Autodesk Inventor part; units mm, degrees
ref_plane "YZ Plane" through (0, 0, 0) normal (1, 0, 0) x (0, 1, 0)
ref_plane "XZ Plane" through (0, 0, 0) normal (0, 1, 0) x (-1, 0, 0)
ref_plane "XY Plane" through (0, 0, 0) normal (0, 0, 1) x (1, 0, 0)
sketch "Skizze1" plane through (0, 0, 0) normal (0, 1, 0) x (-1, 0, 0)
  line L0 (-60, -60) -> (60, -60)
  line L1 (60, -60) -> (60, 60)
  line L2 (60, 60) -> (-60, 60)
  line L3 (-60, 60) -> (-60, -60)
  line L4 (-60, -60) -> (60, 60) construction
  line L5 (60, -60) -> (-60, 60) construction
  point P0 (0, 0)
  dimension "d0" = 120
  dimension "d1" = 120
extrude "Extrusion1" add sketch "Skizze1" along normal blind 25
sketch "Skizze2" plane through (0, 25, 0) normal (0, 1, 0) x (1, 0, 0)
  line L0 (52.5, 52.5) -> (-52.5, 52.5)
  line L1 (-52.5, 52.5) -> (-52.5, -52.5)
  line L2 (-52.5, -52.5) -> (52.5, -52.5)
  line L3 (52.5, -52.5) -> (52.5, 52.5)
  line L4 (52.5, 52.5) -> (-52.5, -52.5) construction
  line L5 (-52.5, 52.5) -> (52.5, -52.5) construction
  point P0 (0, 0)
  dimension "d4" = 105
  dimension "d5" = 105
hole "Bohrung1" at (52.5, 25, 52.5) at (52.5, 25, -52.5) at (-52.5, 25, 52.5) at (-52.5, 25, -52.5) direction (0, -1, 0) diameter 4.3 end through all
sketch "Skizze3" plane through (0, 25, 0) normal (0, 1, 0) x (1, 0, 0)
  circle A0 centre (0, 0) radius 56.5
  dimension "d13" = 113
extrude "Extrusion2" cut sketch "Skizze3" against normal through all
fillet "Rundung1" radius 2 4 edges at (-60, 12.5, 60) (60, 12.5, 60) (-60, 12.5, -60) (60, 12.5, -60)
properties part number "Lüfter80x80"
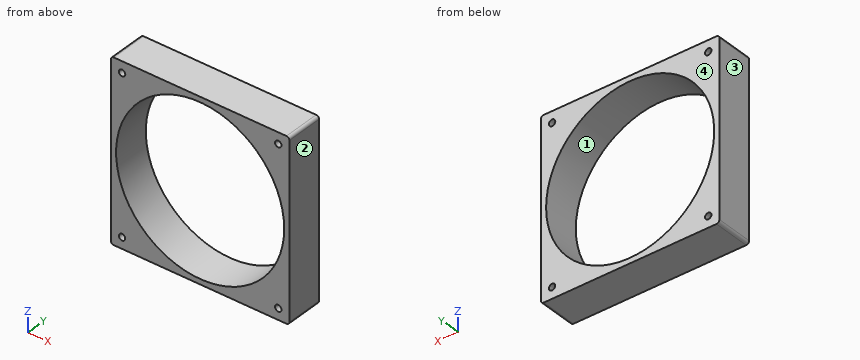
CAD build for the part. Positions are in the model's coordinates, mm. Face numbers are marked on the shaded views. Round coordinates to 2 decimals unless told otherwise and drop trailing zeros. Order: outer loops, then holes, each group sorted by start corner. A loop starts at its lowest first (then second) coordinate and runs counter-clockwise, first axis right, second up. Notation, with made-up numbers: (24, 42.5) - (43, 42.5) arc R13 cw to (43, 49.5) - close; hole circle Ø11 at (74, 72.25). An arc over 180 degrees is marked (long way). Answer in a Markdown table with one row per item. Add a question column.
(1) Band-saw the part on D-D on x = -52.5. List the corners of the cut face in (y, z).
(2) Drop a flat-ended pin along its axis: pin 1 Ø4 at (x, z) = (52.5, -52.5) entering from -Y. Give the stop position or say it passes through.
(3) Probe L1, parallel to X at y = 15.75, z = -1.5; L2, parallel to Z at x = 0, y = 8.75; L3, parallel to X at y = 14.5, z = -52.5. List the from-to ranges inside material, lowest first. Write a range as [from, to].
(4) Band-saw the part on B-B on x = 0. List the corners of the cut face in (y, z).
(5) Band-saw the part on C-C on z = 0. List the corners of the cut face in (x, y), and give its area (3 significant figures).
(6) Band-saw the part on A-A on y = 20.25. List the corners of the cut face in (x, z).
(7) Mould opens along X. For the marked faces 1, 2, 3 and 4 say: +X half, -X half, draft (parallel to the pull), parting line (faces both ways), or undercut.
Data:
| question | item | result |
|---|---|---|
| 1 | outline | (0, -60) - (25, -60) - (25, -54.65) - (0, -54.65) - close; (0, -50.35) - (25, -50.35) - (25, -20.88) - (0, -20.88) - close; (0, 20.88) - (25, 20.88) - (25, 50.35) - (0, 50.35) - close; (0, 54.65) - (25, 54.65) - (25, 60) - (0, 60) - close |
| 2 | pin 1 | passes through |
| 3 | L1 | x = [-60, -56.48], [56.48, 60] |
| 3 | L2 | z = [-60, -56.5], [56.5, 60] |
| 3 | L3 | x = [-60, -54.65], [-50.35, -20.88], [20.88, 50.35], [54.65, 60] |
| 4 | outline | (0, -60) - (25, -60) - (25, -56.5) - (0, -56.5) - close; (0, 56.5) - (25, 56.5) - (25, 60) - (0, 60) - close |
| 5 | outline | (-60, 0) - (-56.5, 0) - (-56.5, 25) - (-60, 25) - close; (56.5, 0) - (60, 0) - (60, 25) - (56.5, 25) - close |
| 5 | area | 175 mm^2 |
| 6 | outline | (-60, -58) arc R2 ccw to (-58, -60) - (58, -60) arc R2 ccw to (60, -58) - (60, 58) arc R2 ccw to (58, 60) - (-58, 60) arc R2 ccw to (-60, 58) - close; hole circle Ø113 at (0, 0); hole circle Ø4.3 at (-52.5, -52.5); hole circle Ø4.3 at (-52.5, 52.5); hole circle Ø4.3 at (52.5, -52.5); hole circle Ø4.3 at (52.5, 52.5) |
| 7 | face 1 | undercut |
| 7 | face 2 | +X half |
| 7 | face 3 | -X half |
| 7 | face 4 | draft |
